from build123d import *

# Parameters (mm, degrees)
SKETCH_1_R      = 3.85
SKETCH_1_R_2    = 1.925
EXTRUDE_1_DEPTH = 1.5


with BuildPart() as part:
    # 草圖1 → 填料-伸長1 (new body)
    with BuildSketch(Plane(origin=(0, 0, 0), x_dir=(0, 0, -1), z_dir=(1, 0, 0))):
        with BuildLine():
            ThreePointArc((111.555989952, -8.572011863), (6.374730125, -10.137132711), (-98.230068302, -21.244930328))
            ThreePointArc((-98.230068302, -21.244930328), (-123.67575498, -2.873316644), (-103.541794939, 21.20204032))
            ThreePointArc((-103.541794939, 21.20204032), (5.082777822, 20.871677912), (113.584507189, 15.696576829))
            ThreePointArc((113.584507189, 15.696576829), (123.827345593, 3.028727453), (112.406990492, -8.588743688))
            ThreePointArc((112.406990492, -8.588743688), (111.981133536, -8.59851924), (111.555989952, -8.572011863))
        make_face()
        with Locations((-102.143981395, 0.133331517)):
            Circle(SKETCH_1_R, mode=Mode.SUBTRACT)
        with Locations((35.001055541, 5.982881827)):
            Circle(SKETCH_1_R_2, mode=Mode.SUBTRACT)
        with Locations((-44.432813653, 4.686665047)):
            Circle(SKETCH_1_R_2, mode=Mode.SUBTRACT)
        with Locations((111.605339346, 3.621333032)):
            Circle(SKETCH_1_R, mode=Mode.SUBTRACT)
    extrude(amount=EXTRUDE_1_DEPTH)


solid = part.part
Check sheet for the modelled part. Datum: model origin and axes. Units: mm. A direction names the side the tool comes from. Give positions to 0.01 mm unless a question says otherwise; leave off trailing zeros. Write each loop counter-clockwise with the first axis right and the second up, starting at its lowest first coordinate (ties: lowest second). Pieces come first, ordered by that corner, then holes. Notation, with made-up numbers: (60, 58) -> (101, 58) arc R25 cw to (101, 79) -> close; hole circle Ø3 at (-15.5, 24.25). An arc over 180 degrees is marked (long way). Write item = value, one per line.
Item 1: Sectioned sample at B-B on z = 89. Record the boundary of the cut face in (x, y).
Output:
outline = (0, -19.88) -> (1.5, -19.88) -> (1.5, 21.44) -> (0, 21.44) -> close
Item 2: Tool access check on faces 4 (the cylindrical face through (0.74, 20.91, -3.56)), 5 (the cylindrical face through (0.74, -10.05, -7.85)), 6 (the cylindrical face through (0.74, 3.79, -107.76)). Record the directions out of +Z, -Z, +X, -X, +Y, -Y that give a thin tool (end or side, any length) a straight path to the whole face; none if there is none.
Output:
face_4 = +X, -X, +Y
face_5 = +X, -X, -Y
face_6 = +X, -X
Item 3: Sectioned sample at C-C on y = -12. Record the boundary of the cut face in (x, z), and give its area (3 significant figures).
Output:
outline = (0, 19.6) -> (1.5, 19.6) -> (1.5, 120.31) -> (0, 120.31) -> close
area = 151 mm^2
Item 4: Release check for a two-part mould opening along Z. For faces 1 (the flat face through (1.5, 5, 26)), 2 (the cylindrical face through (0.74, 6.07, -33.08)), 3 (the cylindrical face through (0.74, 3.278, -123.837)) record: +Z half, -Z half, draft (parallel to the pull), parting line (faces both ways), or undercut.
Output:
face_1 = draft
face_2 = undercut
face_3 = -Z half
Item 5: Scan lines: probe 1 along Z at (x, y) = (0.6, 7); probe 2 along Z at (x, y) = (0.95, 5); probe 3 along Z at (x, y) = (1.1, 3). Record each from-to range of solid material in increasing order. Write a range as from..to.
Output:
probe_1 = -123.37..-113.45, -109.76..-36.64, -33.37..122.59
probe_2 = -123.76..-115.2, -108.01..-36.66, -33.35..42.53, 46.33..123.2
probe_3 = -123.83..-115.4, -107.81..43.51, 45.36..99.57, 104.71..123.6
Item 6: Sectioned sample at A-A on x = 1. Count the separate pieces of the cut face and the enclosed holes in it, and give its area (3 significant figures).
Output:
separate_pieces = 1
enclosed_holes = 4
area = 7,690 mm^2
